The drawing under review shows one solid part. Ordinate dimensions are in mm from its lowest x, y, z. A direction names the side the tool comes from. Give positions to 0.01 mm unless a question says otherwise; leave off trailing zeros. Write each loop counter-clockwise with the first axis right and the second up, starting at its lowest first coordinate (ties: lowest second). Pieces come first, ordered by that corner, then holes. Notation, with made-up numbers: (-31, -31.75) -> (19, -31.75) arc R24 cw to (19, 0.25) -> close; hole circle Ø2 at (69, 7.25). An arc over 180 degrees is marked (long way). Answer as a JSON object with one key per item and string values.
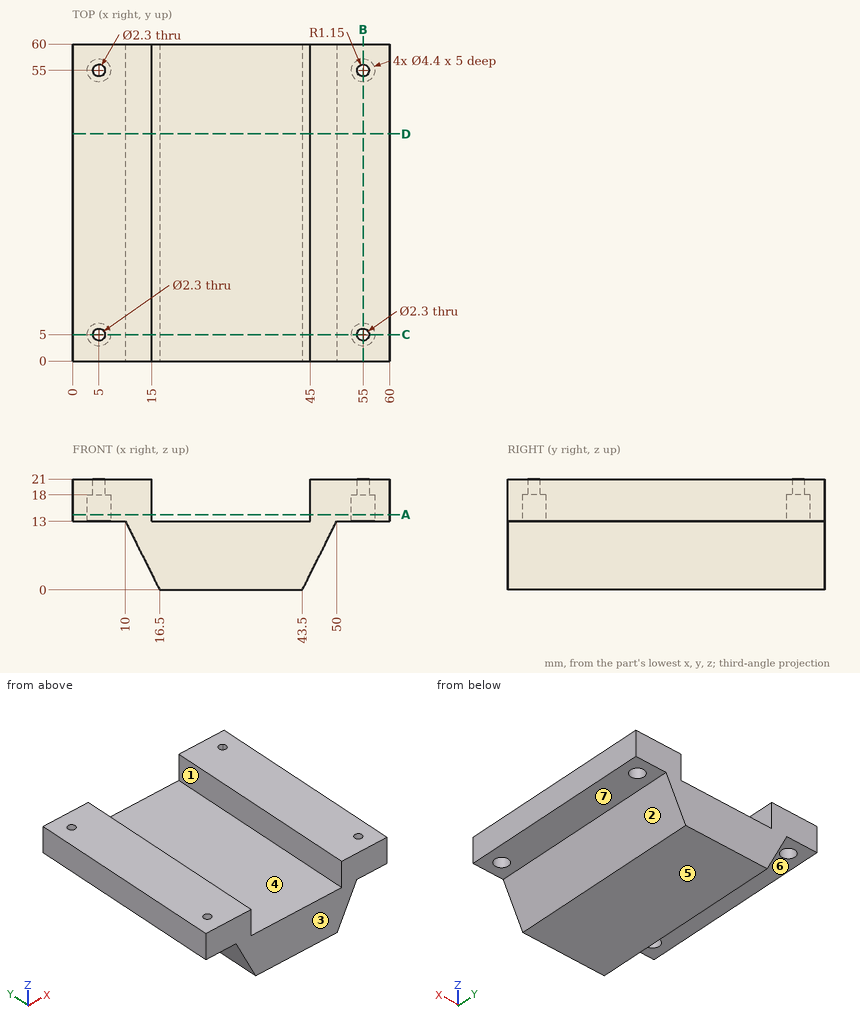
(1) We need section C-C, the plane y = 5. State the section outline as (x, z) points.
Here are the results:
{"outline": "(0, 13) -> (2.8, 13) -> (2.8, 18) -> (3.85, 18) -> (3.85, 21) -> (0, 21) -> close; (6.15, 18) -> (7.2, 18) -> (7.2, 13) -> (10, 13) -> (16.5, 0) -> (43.5, 0) -> (50, 13) -> (52.8, 13) -> (52.8, 18) -> (53.85, 18) -> (53.85, 21) -> (45, 21) -> (45, 13) -> (15, 13) -> (15, 21) -> (6.15, 21) -> close; (56.15, 18) -> (57.2, 18) -> (57.2, 13) -> (60, 13) -> (60, 21) -> (56.15, 21) -> close"}
(2) We need section B-B, the plane x = 55. State the section outline as (y, z) points.
Here are the results:
{"outline": "(0, 13) -> (2.8, 13) -> (2.8, 18) -> (3.85, 18) -> (3.85, 21) -> (0, 21) -> close; (6.15, 18) -> (7.2, 18) -> (7.2, 13) -> (52.8, 13) -> (52.8, 18) -> (53.85, 18) -> (53.85, 21) -> (6.15, 21) -> close; (56.15, 18) -> (57.2, 18) -> (57.2, 13) -> (60, 13) -> (60, 21) -> (56.15, 21) -> close"}
(3) Clearance check with flat-ended pins moving along their axes: pin 1 (3 mm diameter, centred on x = 6.5, y = 20.5, fed in from -Z); pin 2 (10 mm diameter, centred on y = 40, z = 7.5, fed in from -X); pin 3 (1.3 mm diameter, centred on x = 56, y = 54, fed in from -Z). State where each tip first meets the part, or that it passes through.
Here are the results:
{"pin 1": "stops at z = 13", "pin 2": "stops at x = 10.25", "pin 3": "stops at z = 18"}
(4) The part is to be moulded in two halves that separate along X. For the marked faces 1, 2, 3 and 4, say which applies: +X half, -X half, draft (parallel to the pull), parting line (faces both ways), or undercut.
Here are the results:
{"face 1": "undercut", "face 2": "+X half", "face 3": "draft", "face 4": "undercut"}
(5) For line 1 along Y through (x, z) = (5, 16.55); line 2 along X through (y, z) = (16.5, 17.5); line 3 along Y through (x, z) = (55, 20.2), list the stretches that pass through material, from the lowest coordinate up.
Here are the results:
{"line 1": "y = 0 to 2.8, 7.2 to 52.8, 57.2 to 60", "line 2": "x = 0 to 15, 45 to 60", "line 3": "y = 0 to 3.85, 6.15 to 53.85, 56.15 to 60"}
(6) For the marked faces 5, 6 and 7, list the 3-axis set-ups (+Z, -Z, +X, -X, +Y, -Y) from which the entire face can be reached by the end or side of a thin tool; tool diameter is ignored.
Here are the results:
{"face 5": "-Z, +X, -X, +Y, -Y", "face 6": "-Z, -X, +Y, -Y", "face 7": "-Z, +X, +Y, -Y"}
(7) We need section A-A, the plane z = 14.25. State the section outline as (x, y) points.
Here are the results:
{"outline": "(0, 0) -> (15, 0) -> (15, 60) -> (0, 60) -> close; (45, 0) -> (60, 0) -> (60, 60) -> (45, 60) -> close; hole circle Ø4.4 at (5, 5); hole circle Ø4.4 at (5, 55); hole circle Ø4.4 at (55, 5); hole circle Ø4.4 at (55, 55)"}
(8) We need section D-D, the plane y = 43. State the section outline as (x, z) points, then the cut area to 4 significant figures.
Here are the results:
{"outline": "(0, 13) -> (10, 13) -> (16.5, 0) -> (43.5, 0) -> (50, 13) -> (60, 13) -> (60, 21) -> (45, 21) -> (45, 13) -> (15, 13) -> (15, 21) -> (0, 21) -> close", "area": "675.5 mm²"}
